Solid Edge part; units mm, degrees
sketch "Sketch1" plane through (0, 0, 0) normal (0, 0, 1) x (1, 0, 0)
  line L0 (0, 0) -> (17, 0)
  line L1 (17, 0) -> (17, 2)
  line L2 (17, 2) -> (2, 2)
  line L3 (2, 2) -> (2, 17)
  line L4 (2, 17) -> (0, 17)
  line L5 (0, 17) -> (0, 0)
extrude "Protrusion1" add sketch "Sketch1" along normal blind 207
sketch "Sketch2" plane through (8.5, 8.5, 207) normal (0, 0, 1) x (1, 0, 0)
  line L0 (-12, -3.5) -> (-3.5, -3.5)
  line L1 (-3.5, -3.5) -> (-3.5, -12)
  line L2 (-3.5, -12) -> (-12, -12)
  line L3 (-12, -12) -> (-12, -3.5)
  dimension "D1" = 12
  dimension "D2" = 3.5
  dimension "D3" = 12
extrude "ExtrudedProtrusion_2" add sketch "Sketch2" against normal blind 207
sketch "Sketch3" plane through (6.75, 6.75, 0) normal (0, 0, -1) x (0, -1, 0)
  line L0 (-11.0586, -10.6054) -> (14.5586, -10.6054)
  line L1 (14.5586, -10.6054) -> (14.5586, 14.1054)
  line L2 (14.5586, 14.1054) -> (-11.0586, 14.1054)
  line L3 (-11.0586, 14.1054) -> (-11.0586, -10.6054)
extrude "ExtrudedCutout_1" cut sketch "Sketch3" against normal blind 2
hole "Hole1" at (8.5, 0, 202) direction (0, 1, 0) diameter 3 end through all
hole "Hole_2" at (8.5, 0, 7) direction (0, 1, 0) diameter 3 end up to next
hole "Hole_3" at (0, 8.5, 202) direction (1, 0, 0) diameter 3 end through all
hole "Hole_4" at (0, 8.5, 7) direction (1, 0, 0) diameter 3 end through all
fillet "Round_1" radius 1 3 edges at (-3.5, -3.5, 104.5) (-3.5, 5, 104.5) (5, -3.5, 104.5)
Geometry: final body of the model. Coordinates: model frame, mm. A direction names the side the tool comes from. Coordinates: 2 decimals unless noted, no trailing zeros. Loops run counter-clockwise (first coordinate to the right, second up) from the corner with the lowest first, then second, coordinate; pieces in that order, holes last. Notation, with made-up numbers: (-37.75, 54) - (-11.75, 54) arc R16 cw to (-11.75, 75) - close; hole circle Ø11 at (5, 18.25). An arc over 180 degrees is marked (long way). Put each result on its own line as item: value. Start each with the question number.
Q1. Pin query (flat end, axial travel): pin 1 Ø2.5 at (y, z) = (8.5, 202) entering from -X; pin 2 Ø1 at (x, z) = (10.5, 73) entering from -Y; pin 3 Ø4 at (x, z) = (5, 131) entering from +Y; pin 4 Ø1.5 at (x, z) = (13, 23) entering from +Y. Return the tip coordinate at first contact, or that it passes through.
Q2. Line query: line 1 (Z direction, x = 8.5, y = 1.1); line 2 (X direction, y = 0.55, z = 202). Output: solid intervals per line, ascending.
Q3. Set-up query: faces 1 (the flat face through (0, 11, 103)), 2 (the flat face through (11, 0, 103)), 3 (the flat face through (2, 11, 103)). Return all of +Z, -Z, +X, -X, +Y, -Y with unobstructed straight access to the full face (end or side cutting, diameter ignored); none if empty.
Q4. Cut plane A-A, the plane z = 179. Return loops of the section in (x, y), and give its area (3 significant figures).
Filled sheet:
1. pin 1: through
1. pin 2: y = 0
1. pin 3: y = 5
1. pin 4: y = 2
2. line 1: 2 to 5.5, 8.5 to 200.5, 203.5 to 207
2. line 2: -3.5 to 7, 10 to 17
3. face 1: +Z, -Z, -X, +Y
3. face 2: +Z, -Z, +X, -Y
3. face 3: +Z, -Z, +X, +Y
4. outline: (-3.5, -2.5) arc R1 ccw to (-2.5, -3.5) - (4, -3.5) arc R1 ccw to (5, -2.5) - (5, 0) - (17, 0) - (17, 2) - (5, 2) - (5, 5) - (2, 5) - (2, 17) - (0, 17) - (0, 5) - (-2.5, 5) arc R1 ccw to (-3.5, 4) - close
4. area: 120 mm²
